from build123d import *

# Parameters (mm, degrees)
F0_W     = 76.2
F0_H     = 76.2
F1_DEPTH = 19.05


with BuildPart() as f1:
    # F0 (on Front) → F1 (new body)
    with BuildSketch(Plane.XZ):
        Polygon((28.333674, 257.741991), (-301.866326, 257.741991), (-301.866326, -72.458009), (-124.066326, -72.458009), (-124.066326, -250.258009), (206.133674, -250.258009), (206.133674, 79.941991), (28.333674, 79.941991), align=None)
        Polygon((168.033674, -212.158009), (-85.966326, -212.158009), (-85.966326, -72.458009), (28.333674, -72.458009), (28.333674, 41.841991), (168.033674, 41.841991), align=None, mode=Mode.SUBTRACT)
        with Locations((-47.866326, 3.741991)):
            Rectangle(F0_W, F0_H, mode=Mode.SUBTRACT)
        Polygon((-263.766326, -34.358009), (-263.766326, 219.641991), (-9.766326, 219.641991), (-9.766326, 79.941991), (-124.066326, 79.941991), (-124.066326, -34.358009), align=None, mode=Mode.SUBTRACT)
    extrude(amount=F1_DEPTH)


solid = f1.part
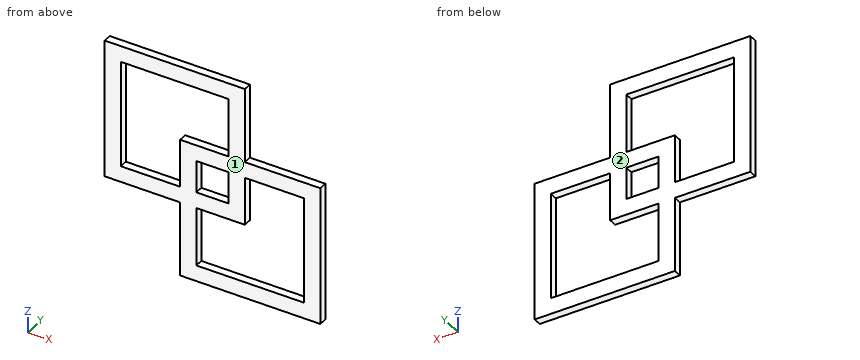
Can you work these out from the model? Positions are in its coordinate system, mm. Face numbers are marked on the shaded views. Round coordinates to 2 decimals unless told otherwise and drop trailing zeros. Loops run counter-clockwise (first coordinate to the right, second up) from the corner with the lowest first, then second, coordinate; pieces in that order, holes last. Notation, with made-up numbers: (87.5, -10.75) - (101.5, -10.75) arc R22 ccw to (101.5, 9.25) - close; hole circle Ø10 at (52, 39). An arc over 180 degrees is marked (long way). Write item = value, one per line. Start each with the question number.
(1) If we section it at C-C (y = -8): Please give me the cut outline in (x, z), and give its area (3 significant figures).
(2) If I drill on probe 1 along Z at (x, y) = (-164, -10.25); probe 2 along X at (y, z) = (-8.5, -200.5); probe 3 along X at (y, z) = (-6, 178), over which ranges is the centre line in solid material (lowest first)? Write a range as [from, to].
(3) If we section it at D-D (z = -150): Please give me the cut outline in (x, y), and give its area (3 significant figures).
(4) If we mould it in two halves opening along Y, with no side actions, what happens to the marked faces 1 and 2? For each: released by +Y, released by -Y, zero draft, split by the parting line, or undercut.
(5) For P1, Ø9.5, axis at y = -12, z = -108, coming from the -X side; P2, Ø9.5, axis at y = -12.5, z = 142, coming from the +X side; P3, Ø9.5, axis at x = -186.5, y = -11.5, coming from the -Z side, each with a flat end and sliding along its axis, tell me the tip position at first contact or that it passes through.
(6) If we section it at B-B (x = 52): Please give me the cut outline in (y, z), and give its area (3 significant figures).
(7) If we section it at A-A (z = 12.5): Please give me the cut outline in (x, y).
Ans:
q1.outline = (-301.87, -72.46) - (-124.07, -72.46) - (-124.07, -250.26) - (206.13, -250.26) - (206.13, 79.94) - (28.33, 79.94) - (28.33, 257.74) - (-301.87, 257.74) - close; hole (-263.77, -34.36) - (-124.07, -34.36) - (-124.07, 79.94) - (-9.77, 79.94) - (-9.77, 219.64) - (-263.77, 219.64) - close; hole (-85.97, -212.16) - (168.03, -212.16) - (168.03, 41.84) - (28.33, 41.84) - (28.33, -72.46) - (-85.97, -72.46) - close; hole (-85.97, -34.36) - (-9.77, -34.36) - (-9.77, 41.84) - (-85.97, 41.84) - close
q1.area = 86,100 mm²
q2.probe_1 = [-72.46, -34.36], [219.64, 257.74]
q2.probe_2 = [-124.07, -85.97], [168.03, 206.13]
q2.probe_3 = [-301.87, -263.77], [-9.77, 28.33]
q3.outline = (-124.07, -19.05) - (-85.97, -19.05) - (-85.97, 0) - (-124.07, 0) - close; (168.03, -19.05) - (206.13, -19.05) - (206.13, 0) - (168.03, 0) - close
q3.area = 1,450 mm²
q4.face_1 = released by -Y
q4.face_2 = released by +Y
q5.P1 = -124.07
q5.P2 = 28.33
q5.P3 = -72.46
q6.outline = (-19.05, -250.26) - (0, -250.26) - (0, -212.16) - (-19.05, -212.16) - close; (-19.05, 41.84) - (0, 41.84) - (0, 79.94) - (-19.05, 79.94) - close
q6.area = 1,450 mm²
q7.outline = (-301.87, -19.05) - (-263.77, -19.05) - (-263.77, 0) - (-301.87, 0) - close; (-124.07, -19.05) - (-85.97, -19.05) - (-85.97, 0) - (-124.07, 0) - close; (-9.77, -19.05) - (28.33, -19.05) - (28.33, 0) - (-9.77, 0) - close; (168.03, -19.05) - (206.13, -19.05) - (206.13, 0) - (168.03, 0) - close
